from build123d import *

# Parameters (mm, degrees)
BOSS_EXTRUDE18_DEPTH = 6
SKETCH22_R           = 12
BOSS_EXTRUDE19_DEPTH = 6
BOSS_EXTRUDE20_DEPTH = 13


with BuildPart() as part:
    # Sketch21 → Boss-Extrude18 (new body)
    with BuildSketch(Plane(origin=(0, 0, 0), x_dir=(1, 0, 0), z_dir=(0, 1, 0))):
        Polygon((0, 55), (-12, 55), (-12, 12), (-55, 12), (-55, 0), (-55, -12), (-12, -12), (-12, -55), (0, -55), (12, -55), (12, -12), (55, -12), (55, 0), (55, 12), (12, 12), (12, 55), align=None)
    extrude(amount=BOSS_EXTRUDE18_DEPTH)

    # Sketch22 → Boss-Extrude19 (add)
    with BuildSketch(Plane(origin=(0, 0, 0), x_dir=(1, 0, 0), z_dir=(0, 1, 0))):
        Circle(SKETCH22_R)
    extrude(amount=BOSS_EXTRUDE19_DEPTH)

    # Sketch16 → Boss-Extrude20 (add)
    with BuildSketch(Plane(origin=(0, 0, 0), x_dir=(1, 0, 0), z_dir=(0, 1, 0))):
        Polygon((-8.834281574, 7.787269814), (9.765718426, 7.787269814), (9.765718426, -21.912730186), (2.765718426, -21.912730186), (2.765718426, -18.912730186), (6.765718426, -18.912730186), (6.765718426, 4.787269814), (-5.834281574, 4.787269814), (-5.834281574, -18.912730186), (-1.834281574, -18.912730186), (-1.834281574, -21.912730186), (-8.834281574, -21.912730186), align=None)
    extrude(amount=BOSS_EXTRUDE20_DEPTH)


solid = part.part
Verification items for the finished model (mm, model axes). A direction names the side the tool comes from. Coordinates: 2 decimals unless noted, no trailing zeros. Order: outer loops, then holes, each group sorted by start corner. A loop starts at its lowest first (then second) coordinate and runs counter-clockwise, first axis right, second up.
Item 1: Depth check by flat-ended pin: pin 1 (1.2 mm diameter, centred on x = 4, y = 8.5, fed in from -Z); pin 2 (1.5 mm diameter, centred on x = -41.5, y = 5.5, fed in from +Z); pin 3 (5 mm diameter, centred on y = 3, z = -27, fed in from +X). Enter the tip coordinate at first touch or a pass-through.
Filled in:
pin 1: stops at z = -7.79
pin 2: stops at z = 12
pin 3: stops at x = 12
Item 2: Section check A-A, the plane y = 1.25. Enter the section's corners in (x, z).
Filled in:
outline: (-55, -12) - (-12, -12) - (-12, -55) - (12, -55) - (12, -12) - (55, -12) - (55, 12) - (12, 12) - (12, 55) - (-12, 55) - (-12, 12) - (-55, 12) - close
Item 3: Material ranges on L1, parallel to X at y = 11.25, z = 10.5; L2, parallel to Z at x = 31, y = 5; L3, parallel to Z at x = -2, y = 12, recorded low to high.
Filled in:
L1: x = -8.83 to -5.83, 6.77 to 9.77
L2: z = -12 to 12
L3: z = -7.79 to -4.79, 18.91 to 21.91
Item 4: Release check for a two-part mould opening along Z. For faces 1 (the face through (34, 3, -12)), 2 (the face through (1, 9, -4.787)), 3 (the face through (1, 0, -1)) record: +Z half, -Z half, draft (parallel to the pull), parting line (faces both ways), or undercut.
Filled in:
face 1: -Z half
face 2: undercut
face 3: draft
Item 5: Section check D-D, the plane z = -35. Enter the section's corners in (x, y), then the cut area to 3 significant figures.
Filled in:
outline: (-12, 0) - (12, 0) - (12, 6) - (-12, 6) - close
area: 144 mm2
Item 6: Section check B-B, the plane z = 5. Enter the section's corners in (x, y).
Filled in:
outline: (-55, 0) - (55, 0) - (55, 6) - (9.77, 6) - (9.77, 13) - (6.77, 13) - (6.77, 6) - (-5.83, 6) - (-5.83, 13) - (-8.83, 13) - (-8.83, 6) - (-55, 6) - close
Item 7: Section check C-C, the plane x = -43.5. Enter the section's corners in (y, z), then the cut area to 3 significant figures.
Filled in:
outline: (0, -12) - (6, -12) - (6, 12) - (0, 12) - close
area: 144 mm2
Item 8: Access from +Z, -Z, +X, -X, +Y, -Y to the whole of each face (thin tool, end or side, straight path). Record for faces 4 (the face through (-4, 9, 18.913)), 5 (the face through (12, 3, 34)), 6 (the face through (-12, 3, -34)).
Filled in:
face 4: +Y
face 5: +Z, +X, +Y, -Y
face 6: -Z, -X, +Y, -Y
